from build123d import *

# Parameters (mm, degrees)
SKETCH_W     = 5.6
SKETCH_H     = 7
PAD_DEPTH    = 4.5
SKETCH001_R  = 2
PAD001_DEPTH = 1.6
SKETCH002_R  = 1
PAD002_DEPTH = 3.3


with BuildPart() as part:
    with BuildSketch(Plane.XY):
        with Locations((196.193, -74.803)):
            Rectangle(SKETCH_W, SKETCH_H)
    extrude(amount=PAD_DEPTH)

    # Sketch001 (on Face2 of Pad) → Pad001 (join)
    with BuildSketch(Plane.YZ.offset(198.993)):
        with Locations((-74.803, 2.25)):
            Circle(SKETCH001_R)
    extrude(amount=PAD001_DEPTH)

    # Sketch002 (on Face8 of Pad001) → Pad002 (join)
    with BuildSketch(Plane.YZ.offset(200.593)):
        with Locations((-74.803, 2.25)):
            Circle(SKETCH002_R)
    extrude(amount=PAD002_DEPTH)


solid = part.part
Read the model definition and answer for the solid it produces. Units are mm, in the model's axes. A direction names the side the tool comes from. Give positions to 0.01 mm unless a question says otherwise; leave off trailing zeros. Write each loop counter-clockwise with the first axis right and the second up, starting at its lowest first coordinate (ties: lowest second). Pieces come first, ordered by that corner, then holes. Notation, with made-up numbers: (55, 35.25) - (77, 35.25) arc R28 cw to (77, 62.25) - close; hole circle Ø4 at (39.5, -38.75). An arc over 180 degrees is marked (long way). Return JSON: item names as keys, results as strings.
Q1. For faces 1 (the face through (200.593, -76, 2)), 2 (the face through (193.393, -75, 2)), determine the directions among +Z, -Z, +X, -X, +Y, -Y from which every point of the face is accessible in a straight line to the end or side of a thin tool.
Reply:
{"face 1": "+X", "face 2": "+Z, -Z, -X, +Y, -Y"}
Q2. Consider line 1 along X through (y, z) = (-77, 0.55); line 2 along X through (y, z) = (-74.5, 0.9); line 3 along Y through (x, z) = (199.5, 2.6). Determine where each line is inside the solid, lowest interval first. Write a range as [from, to].
Reply:
{"line 1": "[193.39, 198.99]", "line 2": "[193.39, 200.59]", "line 3": "[-76.77, -72.83]"}
Q3. A cutting plane is placed at A-A, the plane z = 2.25. Determine the outline of the cut face in (x, y), and give its area (3 significant figures).
Reply:
{"outline": "(193.39, -78.3) - (198.99, -78.3) - (198.99, -76.8) - (200.59, -76.8) - (200.59, -75.8) - (203.89, -75.8) - (203.89, -73.8) - (200.59, -73.8) - (200.59, -72.8) - (198.99, -72.8) - (198.99, -71.3) - (193.39, -71.3) - close", "area": "52.2 mm²"}
Q4. Given P1, Ø2, axis at y = -72.5, z = 1.5, coming from the +X side, flat-ended and moving along its own axis, determine where the tip first touches the part or whether it passes through.
Reply:
{"P1": "x = 200.59"}
Q5. A cutting plane is placed at C-C, the plane x = 202.75. Determine the outline of the cut face in (y, z), and give its area (3 significant figures).
Reply:
{"outline": "circle Ø2 at (-74.8, 2.25)", "area": "3.14 mm²"}
Q6. A cutting plane is placed at D-D, the plane y = -74.25. Determine the outline of the cut face in (x, z).
Reply:
{"outline": "(193.39, 0) - (198.99, 0) - (198.99, 0.33) - (200.59, 0.33) - (200.59, 1.42) - (203.89, 1.42) - (203.89, 3.08) - (200.59, 3.08) - (200.59, 4.17) - (198.99, 4.17) - (198.99, 4.5) - (193.39, 4.5) - close"}
Q7. A cutting plane is placed at B-B, the plane y = -72.25. Determine the outline of the cut face in (x, z), and give its area (3 significant figures).
Reply:
{"outline": "(193.39, 0) - (198.99, 0) - (198.99, 4.5) - (193.39, 4.5) - close", "area": "25.2 mm²"}
